Input: part model. Units: mm. Frame: model coordinates. A direction names the side the tool comes from. Round coordinates to 2 decimals unless told otherwise and drop trailing zeros. Order: outer loops, then holes, each group sorted by start corner. A loop starts at its lowest first (then second) coordinate and runs counter-clockwise, first axis right, second up.
Item 1: Line query: L1, parallel to Z at x = -14, y = 4.5; L2, parallel to Y at x = 36, z = 0; L3, parallel to Y at x = -22, z = 4.5. Output: solid intervals per line, ascending.
Item 2: Reachability of faces 1 (the cylindrical face through (33.4, -5.1, -1.47)), 2 (the cylindrical face through (-26.916, -7.325, 0.134)) from +Z, -Z, +X, -X, +Y, -Y: full face, straight path, thin tool, end or side. Return the list, or none.
Item 3: Cut plane C-C on z = 16. Output: boundary loops of the cut face in (x, y), then the cut area to 3 significant figures.
Item 4: Cut plane B-B on x = -13. Output: boundary loops of the cut face in (y, z), then the cut area to 3 significant figures.
Item 5: Mould query, pull axis Z, two halves, no side actions, for faces 3 (the flat face through (-31.3, 4.191, 2.5)), 4 (the cylindrical face through (10.643, 5.801, 33.797)). Classes: released by +Z, released by -Z, zero draft, split by the parting line, or undercut.
Item 6: First-contact query: pin 1 (8 mm diameter, centred on y = -3, z = -10.5, fed in from +X); pin 2 (1 mm diameter, centred on y = 4, z = -3, fed in from +X); pin 3 (8 mm diameter, centred on y = -3.5, z = 30, fed in from -X). Flat tips, straight axial feed; report the tip coordinate or a pass-through.
Item 7: Cut plane D-D on x = -27.94. Output: boundary loops of the cut face in (y, z) (1 decimal).
Item 8: Cut plane A-A on x = 18. Output: boundary loops of the cut face in (y, z).
```python
from build123d import *

# Parameters (mm, degrees)
SKETCH2_R          = 1.7272
CUT_EXTRUDE1_DEPTH = 55.61
SKETCH3_R          = 35.433
SKETCH3_R_2        = 31.242
CUT_EXTRUDE2_DEPTH = 3.175
SKETCH4_R          = 1.03251
CUT_EXTRUDE3_DEPTH = 3.175
CIRPATTERN1_COUNT  = 9
SKETCH5_R          = 3.175
CUT_EXTRUDE4_DEPTH = 9.525
FILLET1_R          = 1.27


with BuildPart() as part:
    # Sketch1 → Revolve1 (revolve)
    with BuildSketch(Plane.XY, mode=Mode.PRIVATE) as revolve1_sk:
        with BuildLine():
            Line((3.8608, 7.366), (38.1, 7.366))
            Line((38.1, 7.366), (38.1, -8.89))
            Line((38.1, -8.89), (22.6695, -8.89))
            Line((22.6695, -8.89), (22.6695, -7.874))
            Line((22.6695, -7.874), (21.1455, -7.874))
            Line((21.1455, -7.874), (21.1455, -8.89))
            Line((21.1455, -8.89), (10.9855, -8.89))
            Line((10.9855, -8.89), (10.9855, -6.391948453))
            ThreePointArc((10.9855, -6.391948453), (10.570616467, -5.000733157), (9.4615, -4.064))
            Line((9.4615, -4.064), (3.8608, 0))
            Line((3.8608, 0), (3.8608, 7.366))
        make_face()
    revolve(revolve1_sk.sketch.rotate(Axis((0, 101.60464546, 0), (0, 1, 0)), 90), axis=Axis((0, 101.60464546, 0), (0, 1, 0)))

    # Sketch2 → Cut-Extrude1 (cut, through all)
    with BuildSketch(Plane(origin=(0, 0, 0), x_dir=(0, 0, -1), z_dir=(1, 0, 0))):
        with Locations(Location((0, -2.286, 0), (0, 0, 270))):
            Circle(SKETCH2_R)
    extrude(amount=CUT_EXTRUDE1_DEPTH, mode=Mode.SUBTRACT)

    # Sketch3 → Cut-Extrude2 (cut)
    with BuildSketch(Plane(origin=(0, 7.366, 0), x_dir=(1, 0, 0), z_dir=(0, 1, 0))):
        with Locations(Location((0, 0, 0), (0, 0, 270))):
            Circle(SKETCH3_R)
        with Locations(Location((0, 0, 0), (0, 0, 270))):
            Circle(SKETCH3_R_2, mode=Mode.SUBTRACT)
    extrude(amount=-CUT_EXTRUDE2_DEPTH, mode=Mode.SUBTRACT)

    # Sketch4 → Cut-Extrude3 (cut)
    with BuildSketch(Plane(origin=(0, -8.89, 0), x_dir=(-1, 0, 0), z_dir=(0, -1, 0))):
        with Locations(Location((-13.97, 24.196749782, 0), (0, 0, 90))):
            Circle(SKETCH4_R)
    cut_extrude3 = extrude(amount=-CUT_EXTRUDE3_DEPTH, mode=Mode.SUBTRACT)

    # CirPattern1: Cut-Extrude3 ×9 about axis
    cirpattern1_axis = Axis((0, 0, 0), (0, 1, 0))
    for i in range(1, CIRPATTERN1_COUNT):
        add(cut_extrude3.rotate(cirpattern1_axis, i * 360 / CIRPATTERN1_COUNT), mode=Mode.SUBTRACT)

    # Sketch5 → Cut-Extrude4 (cut)
    with BuildSketch(Plane(origin=(38.1, 0, 0), x_dir=(0, 0, -1), z_dir=(1, 0, 0))):
        with Locations((0, -2.286)):
            Circle(SKETCH5_R)
    extrude(amount=-CUT_EXTRUDE4_DEPTH, mode=Mode.SUBTRACT)

    # Fillet1
    fillet1_edges = [part.edges().sort_by_distance(p)[0] for p in [
        (0, 0, 3.8608),
    ]]
    fillet(fillet1_edges, radius=FILLET1_R)


solid = part.part
```
From the geometry:
1. L1: z = -35.43 to -32.55, -27.93 to 27.93, 32.55 to 35.43
1. L2: y = -8.89 to -5.46, 0.89 to 7.37
1. L3: y = -7.87 to 7.37
2. face 1: +X
2. face 2: -Y
3. outline: (-34.58, -8.89) - (-16.06, -8.89) - (-16.06, -7.87) - (-13.83, -7.87) - (-13.83, -8.89) - (13.83, -8.89) - (13.83, -7.87) - (16.06, -7.87) - (16.06, -8.89) - (34.58, -8.89) - (34.58, 7.37) - (31.61, 7.37) - (31.61, 4.19) - (26.83, 4.19) - (26.83, 7.37) - (-26.83, 7.37) - (-26.83, 4.19) - (-31.61, 4.19) - (-31.61, 7.37) - (-34.58, 7.37) - close
3. area: 1,090 mm2
4. outline: (-8.89, -35.81) - (7.37, -35.81) - (7.37, -32.96) - (4.19, -32.96) - (4.19, -28.41) - (7.37, -28.41) - (7.37, 28.41) - (4.19, 28.41) - (4.19, 32.96) - (7.37, 32.96) - (7.37, 35.81) - (-8.89, 35.81) - (-8.89, 18.57) - (-7.87, 18.57) - (-7.87, 16.68) - (-8.89, 16.68) - (-8.89, -16.68) - (-7.87, -16.68) - (-7.87, -18.57) - (-8.89, -18.57) - close
4. area: 1,130 mm2
5. face 3: undercut
5. face 4: undercut
6. pin 1: stops at x = 37.54
6. pin 2: stops at x = 38.02
6. pin 3: stops at x = -27.85
7. outline: (-8.9, -25.9) - (7.4, -25.9) - (7.4, -21.8) - (4.2, -21.8) - (4.2, -14) - (7.4, -14) - (7.4, 14) - (4.2, 14) - (4.2, 21.8) - (7.4, 21.8) - (7.4, 25.9) - (-8.9, 25.9) - (-8.9, 1) - (-5.7, 1) - (-5.7, -1) - (-8.9, -1) - close
8. outline: (-8.89, -33.58) - (7.37, -33.58) - (7.37, -30.52) - (4.19, -30.52) - (4.19, -25.54) - (7.37, -25.54) - (7.37, 25.54) - (4.19, 25.54) - (4.19, 30.52) - (7.37, 30.52) - (7.37, 33.58) - (-8.89, 33.58) - (-8.89, 13.78) - (-7.87, 13.78) - (-7.87, 11.1) - (-8.89, 11.1) - (-8.89, -11.1) - (-7.87, -11.1) - (-7.87, -13.78) - (-8.89, -13.78) - close; hole circle Ø3.45 at (-2.29, 0)
